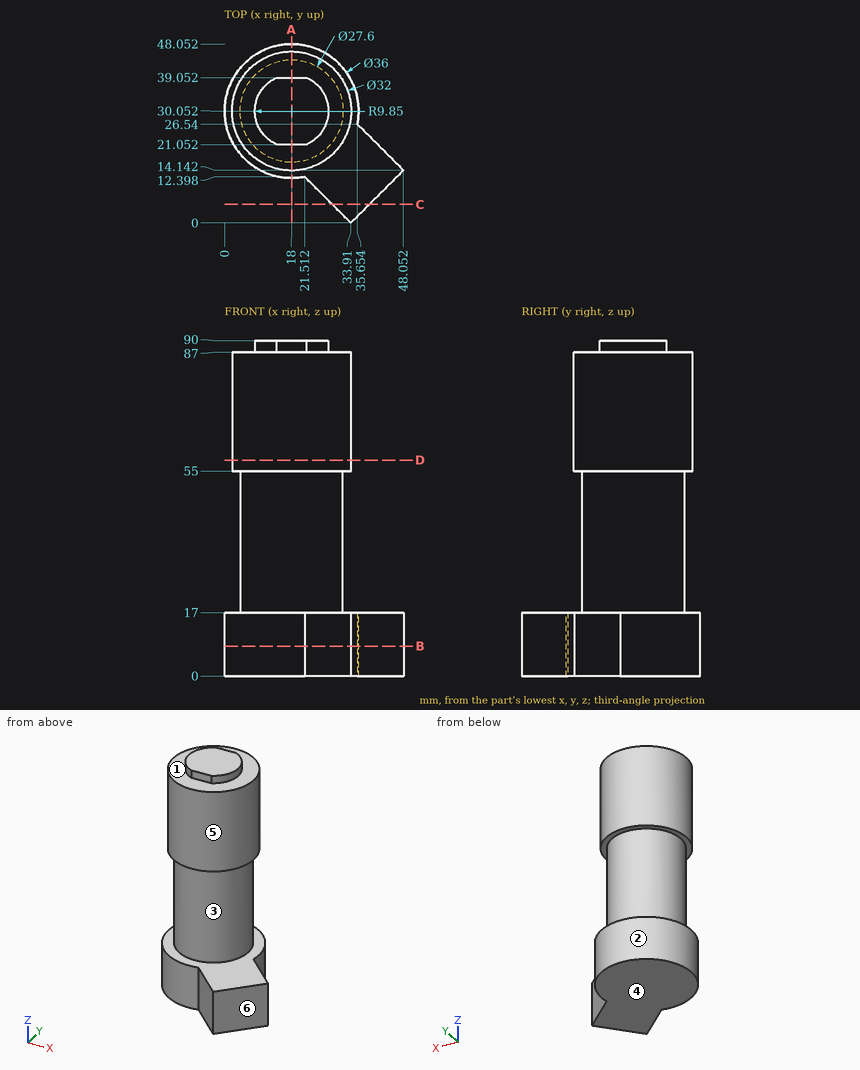
Verification items for this drawing (mm, ordinates from the low corner). A direction names the side the tool comes from. Give positions to 0.01 mm unless a question says otherwise; leave off trailing zeros. Loops run counter-clockwise (first coordinate to the right, second up) from the corner with the lowest first, then second, coordinate; pieces in that order, holes last. Notation, with made-up numbers: M -20.5,53.25 L 34.5,53.25 A22 cw 34.5,60.25 Z; hole C 85,5 d1. An arc over 180 degrees is marked long. Return JSON: item names as keys, results as strings. Group by question number.
1. Cross-section at A-A on x = 18. Record the boundary of the cut face in (y, z), plus the area to 3 significant figures.
2. Go/stop test with flat-tipped pins: pin 1 (12 mm diameter, centred on x = 12.5, z = 77.5, fed in from -Y); pin 2 (8 mm diameter, centred on y = 27, z = 17.5, fed in from +X); pin 3 (1 mm diameter, centred on x = 20.5, y = 27, fed in from -Z); pin 4 (3 mm diameter, centred on y = 31, z = 78.5, fed in from +X). Record where each tip stops, or that it passes through.
3. Mould release check, pull along X, two halves, no side actions. Record for the marked faces 4, 5 and 6: released by +X, released by -X, zero draft, split by the parting line, or undercut.
4. Tool access check on the marked faces 1, 2 and 3. Record the directions out of +Z, -Z, +X, -X, +Y, -Y that give a thin tool (end or side, any length) a straight path to the whole face; none if there is none.
5. Cross-section at B-B on z = 8. Record the boundary of the cut face in (x, y).
6. Cross-section at C-C on y = 5. Record the boundary of the cut face in (x, z).
7. Cross-section at D-D on z = 58. Record the boundary of the cut face in (x, y).
8. Thickness scan on L1, parallel to Z at x = 29, y = 41; L2, parallel to Z at x = 42, y = 18; L3, parallel to Z at x = 22, y = 18.5. Record the ranges inside material, lowest first.
Return value:
{
 "1": {"outline": "M 12.05,0 L 48.05,0 L 48.05,17 L 43.85,17 L 43.85,55 L 46.05,55 L 46.05,87 L 39.05,87 L 39.05,90 L 21.05,90 L 21.05,87 L 14.05,87 L 14.05,55 L 16.25,55 L 16.25,17 L 12.05,17 Z", "area": "2,740 mm^2"},
 "2": {"pin 1": "y = 14.05", "pin 2": "x = 39.16", "pin 3": "z = 0", "pin 4": "x = 34"},
 "3": {"face 4": "zero draft", "face 5": "split by the parting line", "face 6": "released by +X"},
 "4": {"face 1": "+Z", "face 2": "+Z, -Z", "face 3": "none"},
 "5": {"outline": "M 21.51,12.4 L 33.91,0 L 48.05,14.14 L 35.65,26.54 A18 ccw long Z"},
 "6": {"outline": "M 28.91,0 L 38.91,0 L 38.91,17 L 28.91,17 Z"},
 "7": {"outline": "C 18,30.05 d32"},
 "8": {"L1": "0 to 17, 55 to 87", "L2": "0 to 17", "L3": "0 to 87"}
}
